Source: CAD feature listing. Evaluate the final solid. Frame: model axes, mm. A direction names the side the tool comes from. Coordinates: 2 decimals unless noted, no trailing zeros. Loops run counter-clockwise (first coordinate to the right, second up) from the corner with the lowest first, then second, coordinate; pieces in that order, holes last.
Item 1: Line query: probe 1 along Y at (x, z) = (-6, 2); probe 2 along Z at (x, y) = (0, -0.6); probe 3 along Y at (x, z) = (-2.5, 15). Output: solid intervals per line, ascending.
Item 2: Section query D-D, the plane y = -0.75. Return the cut outline in (x, z), then the cut area to 3 significant figures.
Item 3: Section query C-C, the plane y = -5.5. Return the cut outline in (x, z).
Item 4: Section query A-A, the plane x = 0. Return the cut outline in (y, z).
Item 5: Pull-direction query (X, two-part tool) for faces 1 (the cylindrical face through (11.923, -16.26, 3.755)), 2 (the cylindrical face through (-4.336, -8.451, -19.524)), 3 (the flat face through (-3.4, 0, 12.3)); classes: +X half, -X half, draft (parallel to the pull), parting line (faces both ways), or undercut.
Item 6: Pin query (flat end, axial travel): pin 1 Ø7.5 at (x, z) = (-4.5, 3.5) entering from +Y; pin 2 Ø5 at (y, z) = (-4, 5) entering from +X; pin 3 Ø6 at (x, y) = (14, -15) entering from +Z. Return the tip coordinate at first contact, or that it passes through.
Item 7: Reachability of faces 4 (the flat face through (-3.4, -17, 12.3)), 5 (the flat face through (0, -15.5, -3)), 6 (the cylindrical face through (-11.923, -0.74, 3.755)) from +Z, -Z, +X, -X, +Y, -Y: full face, straight path, thin tool, end or side. Return the list, or none.
Item 8: Section query B-B, the plane z = 0. Return the cut outline in (x, y).
```python
from build123d import *

# Parameters (mm, degrees)
F0_R     = 20
F0_R_2   = 1.5
F1_DEPTH = 17
F2_R     = 12.5
F3_DEPTH = 1.5
F4_R     = 12.5
F5_DEPTH = 1.5
F6_R     = 5


with BuildPart() as f1:
    # F0 (on Front) → F1 (new body)
    with BuildSketch(Plane.XZ):
        Circle(F0_R)
        Circle(F0_R_2, mode=Mode.SUBTRACT)
    extrude(amount=F1_DEPTH)

    # F2 (on face) → F3 (cut)
    with BuildSketch(Plane.XZ.offset(17)):
        Circle(F2_R)
    extrude(amount=-F3_DEPTH, mode=Mode.SUBTRACT)

    # F4 (on face) → F5 (cut)
    with BuildSketch(Plane(origin=(0, 0, 0), x_dir=(-1, 0, 0), z_dir=(0, 1, 0))):
        Circle(F4_R)
    extrude(amount=-F5_DEPTH, mode=Mode.SUBTRACT)

    # F6
    f6_edges = [f1.edges().sort_by_distance(p)[0] for p in [
        (-20, 0, 0),
        (-20, -17, 0),
    ]]
    fillet(f6_edges, radius=F6_R)


solid = f1.part
```
Verdict:
1. probe 1: y = -15.5 to -1.5
1. probe 2: z = -17.37 to -12.5, 12.5 to 17.37
1. probe 3: y = -17 to 0
2. outline: circle Ø35.27 at (0, 0); hole circle Ø25 at (0, 0)
2. area: 486 mm2
3. outline: circle Ø40 at (0, 0); hole circle Ø3 at (0, 0)
4. outline: (-17, -15) arc R5 ccw to (-12, -20) - (-5, -20) arc R5 ccw to (0, -15) - (0, -12.5) - (-1.5, -12.5) - (-1.5, -1.5) - (-15.5, -1.5) - (-15.5, -12.5) - (-17, -12.5) - close; (-17, 12.5) - (-15.5, 12.5) - (-15.5, 1.5) - (-1.5, 1.5) - (-1.5, 12.5) - (0, 12.5) - (0, 15) arc R5 ccw to (-5, 20) - (-12, 20) arc R5 ccw to (-17, 15) - close
5. face 1: undercut
5. face 2: parting line
5. face 3: draft
6. pin 1: stops at y = -1.5
6. pin 2: stops at x = 19.82
6. pin 3: stops at z = 16.15
7. face 4: +Z, -Z, +X, -X, -Y
7. face 5: -Y
7. face 6: +Y
8. outline: (-20, -12) arc R5 ccw to (-15, -17) - (-12.5, -17) - (-12.5, -15.5) - (-1.5, -15.5) - (-1.5, -1.5) - (-12.5, -1.5) - (-12.5, 0) - (-15, 0) arc R5 ccw to (-20, -5) - close; (1.5, -15.5) - (12.5, -15.5) - (12.5, -17) - (15, -17) arc R5 ccw to (20, -12) - (20, -5) arc R5 ccw to (15, 0) - (12.5, 0) - (12.5, -1.5) - (1.5, -1.5) - close
